Build history of the part. All positions in model axes, mm. A direction names the side the tool comes from. Coordinates: 2 decimals unless noted, no trailing zeros. Loops run counter-clockwise (first coordinate to the right, second up) from the corner with the lowest first, then second, coordinate; pieces in that order, holes last. Notation, with made-up numbers: (62.25, 21) - (91.25, 21) arc R29 cw to (91.25, 41) - close; hole circle Ø11 at (43, 56.25). An arc over 180 degrees is marked (long way). One line per item, written item: value.
```python
from build123d import *

# Parameters (mm, degrees)
EXTRUDE_THIN1_DEPTH = 20.6375
SKETCH2_R           = 7.14375
CUT_EXTRUDE1_DEPTH  = 109.706083805
SKETCH3_R           = 7.14375
CUT_EXTRUDE2_DEPTH  = 113.354183973


with BuildPart() as part:
    # Sketch1 → Extrude-Thin1 (new, symmetric)
    with BuildSketch(Plane.XY):
        with BuildLine():
            Line((0, 104.775), (0, 7.9375))
            ThreePointArc((0, 7.9375), (2.324839924, 2.324839924), (7.9375, 0))
            Line((7.9375, 0), (41.275, 0))
            Line((41.275, 0), (41.275, 6.35))
            Line((41.275, 6.35), (7.9375, 6.35))
            ThreePointArc((7.9375, 6.35), (6.814967985, 6.814967985), (6.35, 7.9375))
            Line((6.35, 7.9375), (6.35, 104.775))
            Line((6.35, 104.775), (0, 104.775))
        make_face()
    extrude(amount=EXTRUDE_THIN1_DEPTH, both=True)

    # Sketch2 → Cut-Extrude1 (cut, through all)
    with BuildSketch(Plane(origin=(0, 6.35, 0), x_dir=(1, 0, 0), z_dir=(0, 1, 0))):
        with Locations(Location((20.6375, 0, 0), (0, 0, 270))):
            Circle(SKETCH2_R)
    extrude(amount=-CUT_EXTRUDE1_DEPTH, mode=Mode.SUBTRACT)

    # Sketch3 → Cut-Extrude2 (cut, through all)
    with BuildSketch(Plane(origin=(6.35, 0, 0), x_dir=(0, 0, -1), z_dir=(1, 0, 0))):
        with Locations(Location((0, 84.1375, 0), (0, 0, 90))):
            Circle(SKETCH3_R)
        with Locations(Location((0, 36.5125, 0), (0, 0, 90))):
            Circle(SKETCH3_R)
    extrude(amount=-CUT_EXTRUDE2_DEPTH, mode=Mode.SUBTRACT)


solid = part.part
```
Item 1: Cut at C-C, the plane z = 0. Give the number of separate pieces and of enclosed holes in the cut face, then the cut area to 3 significant figures.
Check result:
separate pieces: 4
enclosed holes: 0
area: 602 mm^2
Item 2: Cut at D-D, the plane y = 87.5. Write the cut outline in (x, z).
Check result:
outline: (0, -20.64) - (6.35, -20.64) - (6.35, -6.3) - (0, -6.3) - close; (0, 6.3) - (6.35, 6.3) - (6.35, 20.64) - (0, 20.64) - close
Item 3: Probe probe 1 along X at (y, z) = (67, 11); probe 2 along Y at (x, z) = (6, -3.5) (3 decimals). List the from-to ranges inside material, lowest first. Write a range as from..to.
Check result:
probe 1: x = 0..6.35
probe 2: y = 0.24..30.285, 42.74..77.91, 90.365..104.775
Item 4: Pull direction Y, two halves, no side cores. Call faces 1 (the face through (2.26, 2.39, 0.29)), 2 (the face through (3.219, 35.583, 7.083)), 3 (the face through (29, 6.35, 0)), 4 (the face through (3.219, 90.737, -2.736)): released by +Y, released by -Y, zero draft, split by the parting line, or undercut.
Check result:
face 1: released by -Y
face 2: undercut
face 3: released by +Y
face 4: undercut
Item 5: Tool access for faces 5 (the face through (6.35, 56, 0)), 6 (the face through (28, 0, 0)): list every direction of +Z, -Z, +X, -X, +Y, -Y with a clear straight run to the whole face (end or side of a thin tool).
Check result:
face 5: +Z, -Z, +X, +Y
face 6: +Z, -Z, +X, -X, -Y
Item 6: Drop flat-ended pins along their axis: P1, Ø5, axis at y = 30.5, z = 1, coming from the +X side; P2, Ø2, axis at x = 28, z = 2, coming from the +Y side; P3, Ø13, axis at x = 20.64, z = 0, coming from the +Y side. Give the stop position or say it passes through.
Check result:
P1: stops at x = 6.35
P2: stops at y = 6.35
P3: passes through
Item 7: Cut at B-B, the plane x = 23.5. Write the cut outline in (y, z), then the cut area to 3 significant figures.
Check result:
outline: (0, -20.64) - (6.35, -20.64) - (6.35, -6.55) - (0, -6.55) - close; (0, 6.55) - (6.35, 6.55) - (6.35, 20.64) - (0, 20.64) - close
area: 179 mm^2
